```python
from build123d import *

# Parameters (mm, degrees)
SKETCH1_W           = 200
SKETCH1_H           = 100
SKETCH1_R           = 7.5
BOSS_EXTRUDE1_DEPTH = 20
SKETCH2_R           = 7.5
BOSS_EXTRUDE2_DEPTH = 10


with BuildPart() as part:
    # Sketch1 → Boss-Extrude1 (new body)
    with BuildSketch(Plane(origin=(0, 0, 0), x_dir=(1, 0, 0), z_dir=(0, 1, 0))):
        Rectangle(SKETCH1_W, SKETCH1_H)
        with Locations(Location((-75, 30, 0), (0, 0, 270))):
            Circle(SKETCH1_R, mode=Mode.SUBTRACT)
        with Locations(Location((-75, -30, 0), (0, 0, 270))):
            Circle(SKETCH1_R, mode=Mode.SUBTRACT)
        with Locations(Location((-25, 30, 0), (0, 0, 270))):
            Circle(SKETCH1_R, mode=Mode.SUBTRACT)
        with Locations(Location((-25, -30, 0), (0, 0, 270))):
            Circle(SKETCH1_R, mode=Mode.SUBTRACT)
        with Locations(Location((25, 30, 0), (0, 0, 270))):
            Circle(SKETCH1_R, mode=Mode.SUBTRACT)
        with Locations(Location((25, -30, 0), (0, 0, 270))):
            Circle(SKETCH1_R, mode=Mode.SUBTRACT)
        with Locations(Location((75, 30, 0), (0, 0, 270))):
            Circle(SKETCH1_R, mode=Mode.SUBTRACT)
        with Locations(Location((75, -30, 0), (0, 0, 270))):
            Circle(SKETCH1_R, mode=Mode.SUBTRACT)
    extrude(amount=BOSS_EXTRUDE1_DEPTH)

    # Sketch2 → Boss-Extrude2 (add, symmetric)
    with BuildSketch(Plane.XY):
        with BuildLine():
            Line((-100, 20), (-157.3406431, 60.150350545))
            ThreePointArc((-157.3406431, 60.150350545), (-161.81564798, 79.782621127), (-142.722823192, 86.17916383))
            Line((-142.722823192, 86.17916383), (-14.361406616, 30))
            ThreePointArc((-14.361406616, 30), (0, 37.5), (14.361406616, 30))
            Line((14.361406616, 30), (142.722823192, 86.17916383))
            ThreePointArc((142.722823192, 86.17916383), (161.81564798, 79.782621127), (157.3406431, 60.150350545))
            Line((157.3406431, 60.150350545), (100, 20))
            Line((100, 20), (-100, 20))
        make_face()
        with Locations((-148.736996555, 72.437631209)):
            Circle(SKETCH2_R, mode=Mode.SUBTRACT)
        with Locations(Location((148.736996555, 72.437631209, 0), (0, 0, 180))):
            Circle(SKETCH2_R, mode=Mode.SUBTRACT)
    extrude(amount=BOSS_EXTRUDE2_DEPTH, both=True)


solid = part.part
```
Geometry: final body of the model. Coordinates: model frame, mm. A direction names the side the tool comes from. Give positions to 0.01 mm unless a question says otherwise; leave off trailing zeros. Order: outer loops, then holes, each group sorted by start corner. A loop starts at its lowest first (then second) coordinate and runs counter-clockwise, first axis right, second up. Notation, with made-up numbers: (-11.5, 41.25) -> (-0.5, 41.25) arc R13 ccw to (-0.5, 56.25) -> close; hole circle Ø8 at (-4.5, 89.25). An arc over 180 degrees is marked (long way). Write each question's results on one line, items separated by ' | '. Start each with the question number.
1) Section A-A (z = 34.5). Return loops of the section in (x, y), then the cut area to 3 significant figures.
2) Section B-B (y = 45). Return loops of the section in (x, z), then the cut area to 3 significant figures.
3) First-contact query: pin 1 (5 mm diameter, centred on x = -19.5, z = -23.5, fed in from +Y); pin 2 (16 mm diameter, centred on y = 12, z = 12.5, fed in from -X); pin 3 (13.5 mm diameter, centred on x = -75, z = 30, fed in from +Y); pin 4 (20 mm diameter, centred on x = 70.5, y = 52.5, fed in from +Z). Flat tips, straight axial feed; report the tip coordinate or a pass-through.
4) Section C-C (x = 75). Return loops of the section in (y, z).
5) Section D-D (x = -90). Return loops of the section in (y, z), then the cut area to 3 significant figures.
6) Line query: line 1 (X direction, y = 6, z = -30); line 2 (X direction, y = 34.5, z = 4); line 3 (X direction, y = 19.5, z = 26). Output: solid intervals per line, ascending. Write a range as from..to.
7) Draft query along Z for faces 1 (the cylindrical face through (32.436, 9.86, -30.976)), 2 (the flat face through (-1, 20, 30)), 3 (the flat face through (-1, 10, 50)), 4 (the cylindrical face through (-19.9, 9.9, -35.5)). Return one class per face: pulls with the +Z half, pulls with the -Z half, needs draft (parallel to the pull), parting line crosses it, or undercut.
8) Set-up query: faces 5 (the flat face through (-1, 0, -1)), 6 (the flat face through (-79.441, 58.483, 0.14)), 7 (the flat face through (2, 32, -10)). Return all of +Z, -Z, +X, -X, +Y, -Y with unobstructed straight access to the full face (end or side cutting, diameter ignored); none if empty.
Calculated:
1) outline: (-100, 0) -> (-81, 0) -> (-81, 20) -> (-100, 20) -> close; (-69, 0) -> (-31, 0) -> (-31, 20) -> (-69, 20) -> close; (-19, 0) -> (19, 0) -> (19, 20) -> (-19, 20) -> close; (31, 0) -> (69, 0) -> (69, 20) -> (31, 20) -> close; (81, 0) -> (100, 0) -> (100, 20) -> (81, 20) -> close | area: 3,040 mm2
2) outline: (-135.7, -10) -> (-48.63, -10) -> (-48.63, 10) -> (-135.7, 10) -> close; (48.63, -10) -> (135.7, -10) -> (135.7, 10) -> (48.63, 10) -> close | area: 3,480 mm2
3) pin 1: y = 20 | pin 2: x = -100 | pin 3: through | pin 4: z = 10
4) outline: (0, -50) -> (20, -50) -> (20, -37.5) -> (0, -37.5) -> close; (0, -22.5) -> (20, -22.5) -> (20, -10) -> (56.54, -10) -> (56.54, 10) -> (20, 10) -> (20, 22.5) -> (0, 22.5) -> close; (0, 37.5) -> (20, 37.5) -> (20, 50) -> (0, 50) -> close
5) outline: (0, -50) -> (20, -50) -> (20, -10) -> (63.1, -10) -> (63.1, 10) -> (20, 10) -> (20, 50) -> (0, 50) -> close | area: 2,860 mm2
6) line 1: -100..-82.5, -67.5..-32.5, -17.5..17.5, 32.5..67.5, 82.5..100 | line 2: -120.71..-24.64, -9.8..9.8, 24.64..120.71 | line 3: -100..-81.34, -68.66..-31.34, -18.66..18.66, 31.34..68.66, 81.34..100
7) face 1: undercut | face 2: needs draft | face 3: pulls with the +Z half | face 4: undercut
8) face 5: +Z, -Z, +X, -X, -Y | face 6: +Z, -Z, +Y | face 7: -Z, +X, -X, +Y
